Could you check a few things on this model? Use its own coordinates, in mm. Face numbers are marked on the shaded views. A direction names the side the tool comes from. Coordinates: 2 decimals unless noted, no trailing zeros. Loops run counter-clockwise (first coordinate to the right, second up) from the corner with the lowest first, then second, coordinate; pieces in that order, holes last. Notation, with made-up numbers: (-30, -29) - (19, -29) arc R19 cw to (19, 8) - close; hole circle Ø1 at (71, 11.25). An arc over 180 degrees is marked (long way). One line per question, with ' | ' between items. Start each with the question number.
1. We'd pull the mould along X, two halves only. Please class the marked faces 1 and 2: pulls with the +X half, pulls with the -X half, needs draft (parallel to the pull), parting line crosses it, or undercut.
2. Please list where these lines run through material, in increasing order: L1, parallel to Z at x = 0, y = -7; L2, parallel to X at y = 3, z = -42.5; L3, parallel to Z at x = 144.5, y = -14. Write a range as [from, to].
3. I want a section at A-A, the plane z = -148. Write out the boundary of the cut face in (x, y), then the cut area to 3 significant figures.
4. I want a section at D-D, the plane z = 18.5. Write out the boundary of the cut face in (x, y).
5. Which directions (+Z, -Z, +X, -X, +Y, -Y) give clear straight access to the entire face, cutting with the end or side of a thin tool? Please do the marked faces 3, 4 and 5.
6. I want a section at B-B, the plane x = 0. Write out the boundary of the cut face in (y, z).
7. I want a section at C-C, the plane z = 60.5. Write out the boundary of the cut face in (x, y).
8. I'm going to push flat-ended pins straight in: P1, Ø2, axis at x = -94, y = -4.5, coming from the -Z side; P2, Ø5.5, axis at y = -2.5, z = -154.5, coming from the -X side; P3, Ø10, axis at y = -20, z = 14.5, coming from the -X side. Where does each tip first touch, or does it pass through?
from build123d import *

# Parameters (mm, degrees)
F1_DEPTH = 25.4
F3_START = -20.32
F3_DEPTH = 5.08
F4_W     = 43.18
F4_H     = 203.2
F5_DEPTH = 12.7
F6_W     = 5.08
F6_H     = 203.2
F7_DEPTH = 12.7
F8_R     = 50.8
F9_DEPTH = 25.4


with BuildPart() as f1:
    # F0 (on Front) → F1 (new body)
    with BuildSketch(Plane.XZ):
        Polygon((0, 76.7976452439), (-152.4, 76.7976452439), (-152.4, -126.4023547561), (0, -126.4023547561), (152.4, -126.4023547561), (152.4, 76.7976452439), align=None)
    extrude(amount=F1_DEPTH)

    # F2 (on face) → F3 (join)
    with BuildSketch(Plane.XZ.offset(25.4).offset(F3_START)):
        Polygon((-72.1423849463, -126.4023547561), (-98.4636694193, -126.4023547561), (-98.4636694193, -185.8566617808), (-72.1423849463, -185.6018817267), align=None)
        Polygon((-72.1423849463, -185.6018817267), (-98.4636694193, -185.8566617808), (-91.5363952518, -194.8621189437), (-78.3745795488, -194.8621189437), align=None)
        Polygon((72.1423849463, -126.4023547561), (72.1423849463, -185.6018817267), (98.4636694193, -185.8566617808), (98.4636694193, -126.4023547561), align=None)
        Polygon((98.4636694193, -185.8566617808), (72.1423849463, -185.6018817267), (78.3745795488, -194.8621189437), (91.5363952518, -194.8621189437), align=None)
    extrude(amount=-F3_DEPTH)

    # F4 (on face) → F5 (join)
    with BuildSketch(Plane(origin=(0, 0, 0), x_dir=(-1, 0, 0), z_dir=(0, 1, 0))):
        with Locations((-160.6027390623, -24.8023547561)):
            Rectangle(F4_W, F4_H)
        with Locations((160.6027390623, -24.8023547561)):
            Rectangle(F4_W, F4_H)
    extrude(amount=-F5_DEPTH)

    # F6 (on face) → F7 (join)
    with BuildSketch(Plane(origin=(0, 0, 0), x_dir=(-1, 0, 0), z_dir=(0, 1, 0))):
        with Locations((-179.6527390623, -24.8023547561)):
            Rectangle(F6_W, F6_H)
        with Locations((179.6527390623, -24.8023547561)):
            Rectangle(F6_W, F6_H)
    extrude(amount=F7_DEPTH)

    # F8 (on face) → F9 (cut)
    with BuildSketch(Plane(origin=(0, 0, 0), x_dir=(-1, 0, 0), z_dir=(0, 1, 0))):
        with Locations((0, -8.7385885348)):
            Circle(F8_R)
    extrude(amount=-F9_DEPTH, mode=Mode.SUBTRACT)


solid = f1.part
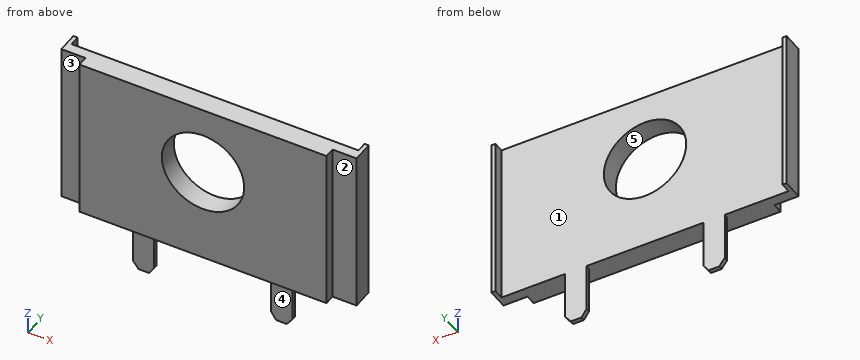
Results are:
1) face 1: undercut | face 2: needs draft
2) L1: z = [-126.4, -59.54], [42.06, 76.8] | L2: x = [-182.19, -177.11], [177.11, 182.19] | L3: z = [-126.4, 76.8]
3) outline: (-98.46, -5.08) - (-72.14, -5.08) - (-72.14, 0) - (-98.46, 0) - close; (72.14, -5.08) - (98.46, -5.08) - (98.46, 0) - (72.14, 0) - close | area: 267 mm2
4) outline: (-182.19, -12.7) - (-152.4, -12.7) - (-152.4, -25.4) - (-42.88, -25.4) - (-42.88, 0) - (-177.11, 0) - (-177.11, 12.7) - (-182.19, 12.7) - close; (42.88, -25.4) - (152.4, -25.4) - (152.4, -12.7) - (182.19, -12.7) - (182.19, 12.7) - (177.11, 12.7) - (177.11, 0) - (42.88, 0) - close
5) face 3: +Z, -Z, -X, -Y | face 4: -Z, +X, -X, -Y | face 5: +Y, -Y
6) outline: (-25.4, -126.4) - (0, -126.4) - (0, -59.54) - (-25.4, -59.54) - close; (-25.4, 42.06) - (0, 42.06) - (0, 76.8) - (-25.4, 76.8) - close
7) outline: (-182.19, -12.7) - (-152.4, -12.7) - (-152.4, -25.4) - (152.4, -25.4) - (152.4, -12.7) - (182.19, -12.7) - (182.19, 12.7) - (177.11, 12.7) - (177.11, 0) - (-177.11, 0) - (-177.11, 12.7) - (-182.19, 12.7) - close
8) P1: stops at z = -192.96 | P2: stops at x = -98.46 | P3: stops at x = -152.4
